Read the model definition and answer for the solid it produces. Units are mm, in the model's axes. A direction names the side the tool comes from. Round coordinates to 2 decimals unless told otherwise and drop trailing zeros. Loops run counter-clockwise (first coordinate to the right, second up) from the corner with the lowest first, then second, coordinate; pieces in that order, holes last. Notation, with made-up numbers: (52, 80.25) - (105, 80.25) arc R33 cw to (105, 117.25) - close; hole circle Ø4 at (29.25, 38.5). An arc over 180 degrees is marked (long way). Answer as CSV lines item,"result".
```python
from build123d import *

# Parameters (mm, degrees)
BOSS_EXTRUDE1_DEPTH = 25
FILLET1_R           = 6
BOSS_EXTRUDE2_DEPTH = 25
FILLET2_R           = 4


with BuildPart() as part:
    # Sketch2 → Boss-Extrude1 (new body)
    with BuildSketch(Plane.XY):
        Polygon((-63, 0), (-60, 0), (-60, -60), (60, -60), (60, 0), (63, 0), (63, -63), (-63, -63), align=None)
    extrude(amount=BOSS_EXTRUDE1_DEPTH)

    # Fillet1
    fillet1_edges = [part.edges().sort_by_distance(p)[0] for p in [
        (-60, -60, 12.5),
        (60, -60, 12.5),
    ]]
    fillet(fillet1_edges, radius=FILLET1_R)

    # Sketch3 → Boss-Extrude2 (add)
    with BuildSketch(Plane(origin=(0, 0, 0), x_dir=(-1, 0, 0), z_dir=(0, 0, -1))):
        Polygon((63, -63), (63, 0), (56.5, 0), (56.5, -56.5), (-56.5, -56.5), (-56.5, 0), (-63, 0), (-63, -63), align=None)
    extrude(amount=BOSS_EXTRUDE2_DEPTH)

    # Fillet2
    fillet2_edges = [part.edges().sort_by_distance(p)[0] for p in [
        (-56.5, -56.5, -12.5),
        (56.5, -56.5, -12.5),
    ]]
    fillet(fillet2_edges, radius=FILLET2_R)


solid = part.part
```
1) A cutting plane is placed at C-C, the plane x = 13. Determine the outline of the cut face in (y, z).
Entries:
outline,"(-63, -25) - (-56.5, -25) - (-56.5, 0) - (-60, 0) - (-60, 25) - (-63, 25) - close"
2) A cutting plane is placed at D-D, the plane z = -6.5. Determine the outline of the cut face in (x, y).
Entries:
outline,"(-63, -63) - (63, -63) - (63, 0) - (56.5, 0) - (56.5, -52.5) arc R4 cw to (52.5, -56.5) - (-52.5, -56.5) arc R4 cw to (-56.5, -52.5) - (-56.5, 0) - (-63, 0) - close"
3) A cutting plane is placed at B-B, the plane z = 7.5. Determine the outline of the cut face in (x, y).
Entries:
outline,"(-63, -63) - (63, -63) - (63, 0) - (60, 0) - (60, -54) arc R6 cw to (54, -60) - (-54, -60) arc R6 cw to (-60, -54) - (-60, 0) - (-63, 0) - close"
4) A cutting plane is placed at A-A, the plane y = -15.5. Determine the outline of the cut face in (x, z).
Entries:
outline,"(-63, -25) - (-56.5, -25) - (-56.5, 0) - (-60, 0) - (-60, 25) - (-63, 25) - close; (56.5, -25) - (63, -25) - (63, 25) - (60, 25) - (60, 0) - (56.5, 0) - close"
5) Find the intervals of material crossed by line 1 (X direction, y = -19, z = 17); line 2 (X direction, y = -22, z = -2); line 3 (Y direction, x = 13, z = 3), in increasing order.
Entries:
line 1,"x = -63 to -60, 60 to 63"
line 2,"x = -63 to -56.5, 56.5 to 63"
line 3,"y = -63 to -60"
6) The mould has two halves that part along X. Classify faces 1 (the face through (-60, -27, 12)), 2 (the face through (0, -57, -25)), 3 (the face through (-63, -32, 0)): pulls with the +X half, pulls with the -X half, needs draft (parallel to the pull), parting line crosses it, or undercut.
Entries:
face 1,"undercut"
face 2,"needs draft"
face 3,"pulls with the -X half"
7) Each of these flat-tipped pins is pushed along its axis until it touches: P1, Ø7.5, axis at x = -19.5, z = -9.5, coming from the +Y side; P2, Ø12.5, axis at x = -20.5, z = 11, coming from the +Y side. Where does it stop, or does it pass through?
Entries:
P1,"stops at y = -56.5"
P2,"stops at y = -60"
8) A tool of negligible diameter and unlimited length cuts with its end or side. For faces 4 (the face through (1, -63, 0)), 5 (the face through (55.297, -55.359, -12.675)), 6 (the face through (0, -57, 0)), from which of +Z, -Z, +X, -X, +Y, -Y can it reach the whole face along a straight path? Write none if from no direction.
Entries:
face 4,"+Z, -Z, +X, -X, -Y"
face 5,"+Z, -Z, +Y"
face 6,"+Z, +Y"
